Autodesk Inventor part; units mm, degrees
ref_plane "YZ Plane" through (0, 0, 0) normal (1, 0, 0) x (0, 1, 0)
ref_plane "XZ Plane" through (0, 0, 0) normal (0, 1, 0) x (-1, 0, 0)
ref_plane "XY Plane" through (0, 0, 0) normal (0, 0, 1) x (1, 0, 0)
sketch "Sketch4" plane through (0, 0, 0) normal (0, 0, 1) x (1, 0, 0)
  line L0 (-14.75, 18) -> (14.7494, 18)
  line L1 (14.7494, 18) -> (14.7494, -10.2)
  line L2 (14.7494, -10.2) -> (-14.75, -10.2)
  line L3 (-14.75, -10.2) -> (-14.75, 18)
  point P0 (0, 0)
  dimension "d24" = 28.2
  dimension "WIDTH" = 29.4994
  dimension "d26" = 14.75
  dimension "d28" = 10.2
extrude "Extrusion3" add sketch "Sketch4" against normal blind 6.4
sketch "Sketch5" plane through (0, 0, 0) normal (0, 0, 1) x (1, 0, 0)
  line L0 (-14.75, -10.2) -> (14.7494, -10.2)
  line L1 (14.7494, -10.2) -> (14.7494, 0)
  line L2 (14.7494, 0) -> (-14.75, 0)
  line L3 (-14.75, 0) -> (-14.75, -10.2)
  line L4 (-14.75, 18) -> (-14.75, -10.2)
  line L5 (-14.75, -10.2) -> (14.7494, -10.2)
  line L6 (14.7494, -10.2) -> (14.7494, 18)
  point P0 (0, 0)
  dimension "d31" = 0
  dimension "d32" = 0
  dimension "d33" = 0
  dimension "d34" = 0
extrude "Extrusion4" add sketch "Sketch5" along normal blind 27.4
sketch "Sketch7" plane through (-14.75, -10.2, -6.4) normal (0, -1, 0) x (1, 0, 0)
  circle A0 centre (14.7497, 19.05) radius 12.8397
  line L0 (29.4994, 33.8) -> (29.4994, 0)
  line L1 (0, 33.8) -> (29.4994, 33.8)
  line L2 (29.4994, 0) -> (0, 0)
  dimension "PILOT_HOLE" = 25.6794
  dimension "d201" = 19.05
  dimension "d202" = 14.7497
sketch "Sketch9" plane through (0, 0, -6.4) normal (0, 0, -1) x (-1, 0, 0)
  line L0 (14.75, 18) -> (-14.7494, 18)
  line L1 (14.75, 0) -> (-14.7494, 0)
  line L2 (0, 6.25) -> (0, 11.75) construction
  line L3 (2.25, 6.25) -> (2.25, 11.75)
  line L4 (-2.25, 11.75) -> (-2.25, 6.25)
  arc A0 (-2.25, 6.25) -> (2.25, 6.25) centre (0, 6.25) ccw
  arc A1 (2.25, 11.75) -> (-2.25, 11.75) centre (0, 11.75) ccw
  line L5 (5.498, 9) -> (4.502, 9) construction
  line L6 (5.498, 10.05) -> (4.502, 10.05)
  line L7 (4.502, 7.95) -> (5.498, 7.95)
  arc A2 (5.498, 7.95) -> (5.498, 10.05) centre (5.498, 9) ccw
  arc A3 (4.502, 10.05) -> (4.502, 7.95) centre (4.502, 9) ccw
  point P0 (0, 0)
  point P1 (-5, 9)
  point P2 (0, 9)
  point P3 (5, 9)
  dimension "d183" = 18
  dimension "d185" = 2.25
  dimension "d186" = 5.5
  dimension "d187" = 0
  dimension "d188" = 9
  dimension "d189" = 1.05
  dimension "d190" = 0.996
  dimension "d191" = 0
  dimension "d192" = 5
extrude "Extrusion6" cut sketch "Sketch9" against normal blind 2.1 contours A2 L7 A3 L6
hole "Hole3" at (5, 9, -6.4) direction (0, 0, 1) diameter 2.1 depth 2.1
extrude "Extrusion7" cut sketch "Sketch7" against normal blind 9.2
sketch "Sketch10" plane through (-0.0003, -1, 12.65) normal (0, -1, 0) x (1, 0, 0)
  circle A0 centre (0, 0) radius 11.85
  circle A1 centre (0, 0) radius 12.8397
  point P0 (0.0003, -12.65)
  point P1 (14.75, 3.9316)
  point P2 (-3.9316, -14.75)
  point P3 (5.6018, -14.2)
  point P4 (-7.6497, 13.2099)
  point P5 (-13.2099, 7.6497)
  point P6 (3.9316, -14.75)
  dimension "d96" = 0
  dimension "d97" = 0
  dimension "d98" = 23.7
extrude "Extrusion8" cut sketch "Sketch10" against normal through all contours A0
extrude "Extrusion9" cut sketch "Sketch9" against normal blind 4.386 contours A0 L4 A1 L3
sketch "Sketch11" plane through (0, 0, -2.014) normal (0, 0, -1) x (-1, 0, 0)
  arc A0 (4, 11.75) -> (-4, 11.75) centre (0, 11.75) ccw
  arc A1 (-4, 6.25) -> (4, 6.25) centre (0, 6.25) ccw
  line L0 (-4, 11.75) -> (-4, 6.25)
  line L1 (4, 6.25) -> (4, 11.75)
  point P0 (0, 0)
  point P1 (0, 9)
  dimension "d136" = 8
  dimension "d137" = 8
  dimension "d138" = 0
  dimension "d139" = 5.5
  dimension "d140" = 0
  dimension "d141" = 2.75
  dimension "d142" = 9
extrude "Extrusion10" cut sketch "Sketch11" against normal through all
chamfer "Chamfer10" distance 1 angle 45 4 edges at (14.7494, -5.1, 27.4) (-14.75, -5.1, 27.4) (14.7494, 18, -3.2) (-14.75, 18, -3.2)
sketch "Sketch13" plane through (-13.75, 18, 0) normal (0, 1, 0) x (1, 0, 0)
  circle A0 centre (13.75, 18.75) radius 12.7
  point P0 (13.75, 0)
  dimension "d196" = 0
  dimension "d197" = 25.4
  dimension "d198" = 18.75
extrude "Extrusion11" cut sketch "Sketch13" against normal up to surface (28.2 mm away)
equation "\"TOLERANCE\" = 0.05"
equation "\"BEAM_HEIGHT\" = 19.05"
properties part number "ADAPTER_SM1"
Verification items for the finished model (mm, model axes). A direction names the side the tool comes from. Coordinates: 2 decimals unless noted, no trailing zeros. Write each loop counter-clockwise with the first axis right and the second up, starting at its lowest first coordinate (ties: lowest second). Pieces come first, ordered by that corner, then holes. Notation, with made-up numbers: (-35.5, 86) - (11.5, 86) arc R27 ccw to (11.5, 115) - close; hole circle Ø11 at (87.5, 25). An arc over 180 degrees is marked (long way). One line per question, with ' | ' between items. Start each with the question number.
1. Draft check along X on faces 1 (the flat face through (2.25, 9, -4)), 2 (the flat face through (14.24, -5.03, 26.91)), 3 (the flat face through (0, -10.2, -1)). Enter one of: released by +X, released by -X, zero draft, split by the parting line, or undercut.
2. Section check C-C (x = 0). Enter the section's corners in (y, z).
3. Access from +Z, -Z, +X, -X, +Y, -Y to the whole of each face (thin tool, end or side, straight path). Record for faces 4 (the flat face through (-5, 10.05, -5)), 5 (the flat face through (4, -1, 1)), 6 (the cylindrical face through (0.09, 2.25, -1.02)), 7 (the flat face through (-2.25, 9, -4)).
4. Material ranges on line 1 along X through (y, z) = (9, -5.8); line 2 along X through (y, z) = (11, -0.5); line 3 along Y through (x, z) = (5, -5.8), recorded low to high.
5. Section check B-B (y = -6.75). Enter the section's corners in (x, z), plus the area to 3 significant figures.
6. Section check D-D (y = 9). Enter the section's corners in (x, z).
7. Gauge pin test, flat ends, axial feed: P1, Ø1.9, axis at x = 5, y = 9, coming from the -Z side; P2, Ø6, axis at x = 7, z = 16.5, coming from the +Y side; P3, Ø9, axis at x = -3, y = 6, coming from the +Z side; P4, Ø13.5, axis at x = 3.5, z = 19, coming from the +Y side. Record the tip position at first contact, or that the pin passes through.
8. Section check A-A (z = 12.65). Enter the section's corners in (x, y), plus the area to 3 significant figures.
Computed values:
1) face 1: undercut | face 2: released by +X | face 3: zero draft
2) outline: (-10.2, -6.05) - (4, -6.05) - (4, -2.01) - (2.25, -2.01) - (2.25, 0) - (0, 0) - (0, 0.8) - (-1, 0.8) - (-1, -0.19) - (-10.2, -0.19) - close; (-10.2, 25.49) - (-1, 25.49) - (-1, 24.5) - (0, 24.5) - (0, 27.4) - (-10.2, 27.4) - close; (14, -6.05) - (18, -6.05) - (18, 0) - (15.75, 0) - (15.75, -2.01) - (14, -2.01) - close
3) face 4: -Z | face 5: -Y | face 6: +Z | face 7: +Z, -Z
4) line 1: -14.75 to -6.55, -3.45 to -2.25, 2.25 to 3.95, 6.05 to 14.75 | line 2: -14.75 to -4, 4 to 14.75 | line 3: -10.2 to 7.95, 10.05 to 18
5) outline: (-14.75, -6.4) - (-2.96, -6.4) arc R12.7 cw to (2.96, -6.4) - (14.75, -6.4) - (14.75, 26.4) - (13.75, 27.4) - (-13.75, 27.4) - (-14.75, 26.4) - close; hole circle Ø25.68 at (0, 12.65) | area: 477 mm²
6) outline: (-14.75, -6.4) - (-6.55, -6.4) - (-6.55, -4.3) - (-3.45, -4.3) - (-3.45, -6.4) - (-2.96, -6.4) arc R12.7 cw to (-2.25, -6.25) - (-2.25, -2.01) - (-4, -2.01) - (-4, 0) - (-14.75, 0) - close; (2.25, -6.25) arc R12.7 cw to (2.96, -6.4) - (3.95, -6.4) - (3.95, -4.3) - (6.05, -4.3) - (6.05, -6.4) - (14.75, -6.4) - (14.75, 0) - (4, 0) - (4, -2.01) - (2.25, -2.01) - close
7) P1: z = -4.3 | P2: through | P3: z = 0 | P4: y = 0
8) outline: (-14.75, -10.2) - (-12.84, -10.2) - (-12.84, -1) - (-11.85, -1) - (-11.85, 0) - (-14.75, 0) - close; (11.85, -1) - (12.84, -1) - (12.84, -10.2) - (14.75, -10.2) - (14.75, 0) - (11.85, 0) - close | area: 40.9 mm²
